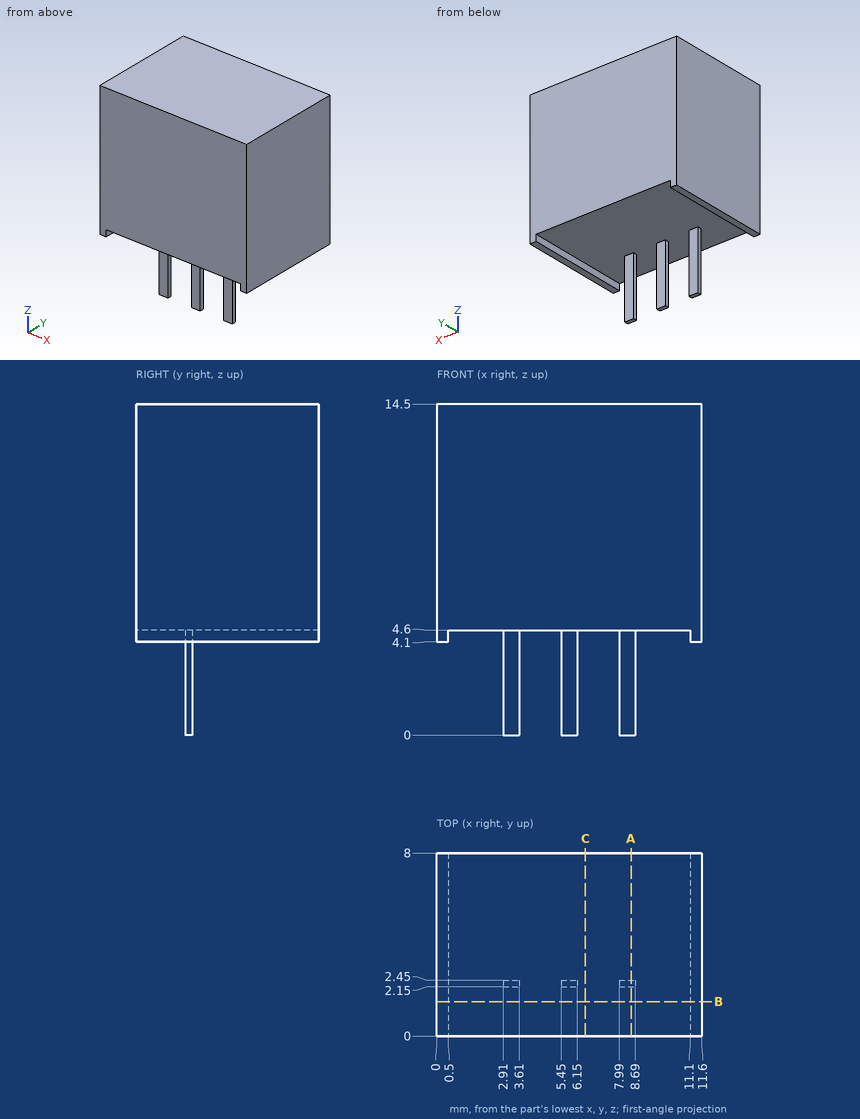
Geometry: see drawing. Coordinates: mm, zero at the bounding-box minimum. Give positions to 0.01 mm unless a question says otherwise; leave off trailing zeros. Loops run counter-clockwise (first coordinate to the right, second up) from the corner with the lowest first, then second, coordinate; pieces in that order, holes last. Notation, with made-up numbers: M 88,5.25 L 118,5.25 A18 cw 118,26.25 Z; hole C -2,-24.5 d1. An arc over 180 degrees is marked long. Answer as CSV lines item,"result". Start each with the question number.
1. Section C-C on x = 6.5. Return loops of the section in (y, z).
2. Section B-B on y = 1.5. Return loops of the section in (x, z).
3. Section A-A on x = 8.5. Return loops of the section in (y, z), plus the area to 3 significant figures.
4. Line query: L1, parallel to Z at x = 9.25, y = 5.5; L2, parallel to X at y = 6.5, z = 4.25. Output: solid intervals per line, ascending.
5. Pin query (flat end, axial travel): P1, Ø0.6, axis at x = 8.5, z = 2.5, coming from the -Y side; P2, Ø0.6, axis at x = 3, z = 2, coming from the +Y side; P3, Ø1.5, axis at x = 2, y = 6.5, coming from the -Z side. Return the tip coordinate at first contact, or that it passes through.
Computed values:
1,outline,"M 0,4.6 L 8,4.6 L 8,14.5 L 0,14.5 Z"
2,outline,"M 0,4.1 L 0.5,4.1 L 0.5,4.6 L 11.1,4.6 L 11.1,4.1 L 11.6,4.1 L 11.6,14.5 L 0,14.5 Z"
3,outline,"M 0,4.6 L 2.15,4.6 L 2.15,0 L 2.45,0 L 2.45,4.6 L 8,4.6 L 8,14.5 L 0,14.5 Z"
3,area,"80.6 mm²"
4,L1,"z = 4.6 to 14.5"
4,L2,"x = 0 to 0.5, 11.1 to 11.6"
5,P1,"stops at y = 2.15"
5,P2,"stops at y = 2.45"
5,P3,"stops at z = 4.6"
